```python
from build123d import *

# Parameters (mm, degrees)
F0_R     = 12.7
F1_DEPTH = 12.7
F2_DEPTH = 304.8


with BuildPart() as f1:
    # F0 (on Front) → F1 (new body)
    with BuildSketch(Plane.XZ):
        with BuildLine():
            Line((13.385539, -79.367668), (67.267937, 44.197556))
            ThreePointArc((67.267937, 44.197556), (66.698178, 49.245503), (62.041647, 51.276051))
            Line((62.041647, 51.276051), (-71.910175, 36.156965))
            ThreePointArc((-71.910175, 36.156965), (-75.996946, 33.139565), (-75.427186, 28.091617))
            Line((-75.427186, 28.091617), (4.642237, -80.35452))
            ThreePointArc((4.642237, -80.35452), (9.298768, -82.385068), (13.385539, -79.367668))
        make_face()
        Circle(F0_R, mode=Mode.SUBTRACT)
    extrude(amount=F1_DEPTH)

    # F0 (on Front) → F2 (join)
    with BuildSketch(Plane.XZ):
        Circle(F0_R)
    extrude(amount=F2_DEPTH)


solid = f1.part
```
CAD build for the part. Positions are in the model's coordinates, mm. A direction names the side the tool comes from. Coordinates: 2 decimals unless noted, no trailing zeros. Write each loop counter-clockwise with the first axis right and the second up, starting at its lowest first coordinate (ties: lowest second). Pieces come first, ordered by that corner, then holes.
(1) Drill centre lines: probe 1 along Y at (x, z) = (-66, 18); probe 2 along X at (y, z) = (-91, 7); probe 3 along Z at (x, y) = (-2, -129). Where is each one in solid material? Low to high.
(2) Cut at A-A, the plane y = -115.5. List the corners of the cut face in (x, z), and give its area (3 significant figures).
(3) Cut at B-B, the plane z = -7. List the corners of the cut face in (x, y), and give its area (3 significant figures).
(4) Flat gauge pins, fed straight in: pin 1 (1 mm diameter, centred on x = 12.5, z = 35, fed in from -Y); pin 2 (10 mm diameter, centred on y = -117.5, z = -12.5, fed in from +X). Where does each tip first touch, or does it go through?
(5) 3-axis set-ups, long thin cutter, end or side, ignore diameter. For faces 1 (the face through (39.95, -6.26, -18.45)), 2 (the face through (-2.75, -156.71, -12.4)): which of +Z, -Z, +X, -X, +Y, -Y reach the whole face in a straight line?
(6) Cut at D-D, the plane z = -33. List the corners of the cut face in (x, y), and give its area (3 significant figures).
(7) Cut at C-C, the plane x = 0. List the corners of the cut face in (y, z).
Geometry says:
1. probe 1: y = -12.7 to 0
1. probe 2: x = -10.6 to 10.6
1. probe 3: z = -12.54 to 12.54
2. outline: circle Ø25.4 at (0, 0)
2. area: 507 mm2
3. outline: (-49.52, -12.7) - (-10.6, -12.7) - (-10.6, -304.8) - (10.6, -304.8) - (10.6, -12.7) - (44.94, -12.7) - (44.94, 0) - (-49.52, 0) - close
3. area: 7,390 mm2
4. pin 1: stops at y = -12.7
4. pin 2: stops at x = 10.25
5. face 1: -Z, +X, +Y, -Y
5. face 2: -Y
6. outline: (-30.32, -12.7) - (33.6, -12.7) - (33.6, 0) - (-30.32, 0) - close
6. area: 812 mm2
7. outline: (-304.8, -12.7) - (-12.7, -12.7) - (-12.7, -74.07) - (0, -74.07) - (0, 44.27) - (-12.7, 44.27) - (-12.7, 12.7) - (-304.8, 12.7) - close
